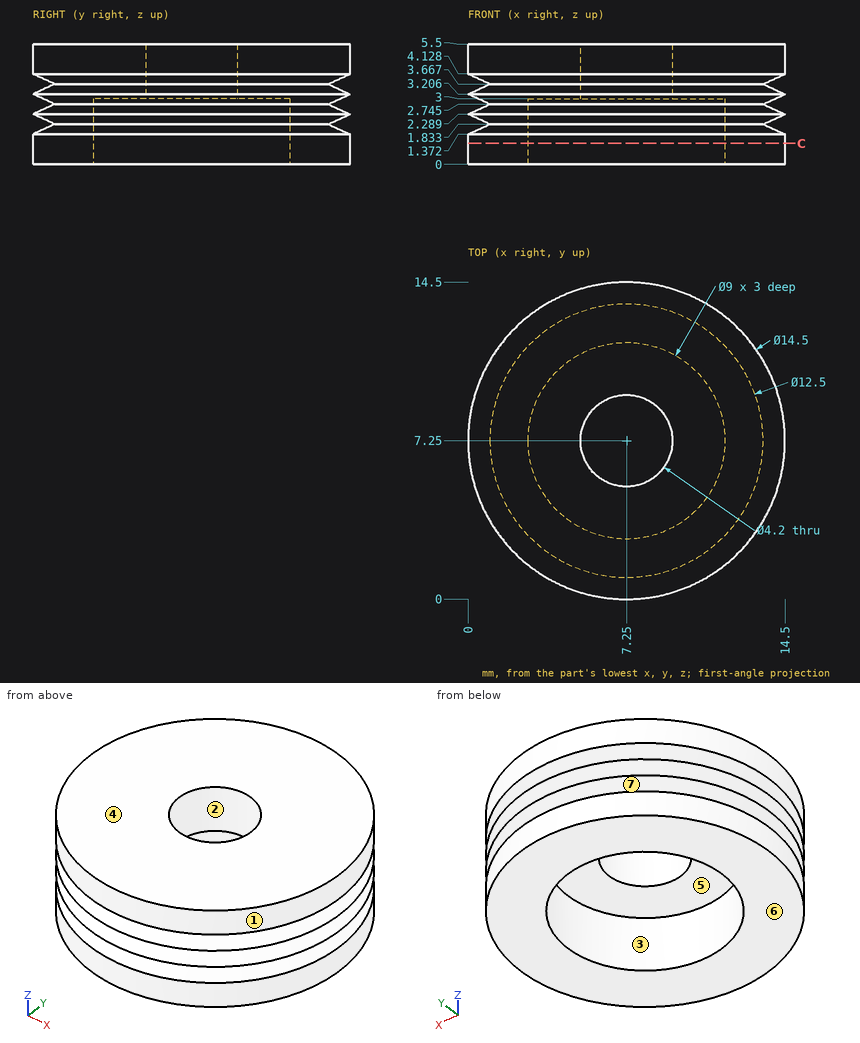
For this review, use the dimensioned drawing (mm, ordinates from the lowest corner) and the shaded views. A direction names the side the tool comes from. Give positions to 0.01 mm unless a question says otherwise; leave off trailing zeros. Order: outer loops, then holes, each group sorted by start corner. A loop starts at its lowest first (then second) coordinate and runs counter-clockwise, first axis right, second up. Notation, with made-up numbers: M 39,27 L 83,27 A23 ccw 83,52 Z; hole C 76.5,63.5 d7. An arc over 180 degrees is marked long. Use one line per item in the form item = value. Start each with the question number.
Item 1: The part is to be moulded in two halves that separate along Y. For the marked faces 1, 2, 3 and 4, say which applies: pulls with the +Y half, pulls with the -Y half, needs draft (parallel to the pull), parting line crosses it, or undercut.
Item 2: Insertion check: pin 1 Ø3 at (x, y) = (2, 3) entering from -Z; pin 2 Ø1.5 at (y, z) = (13, 1.5) entering from -X; pin 3 Ø2.5 at (x, y) = (7, 8.5) entering from -Z. Each pin has a flat end and moves straight along its axis. Give the tip position at first contact, or say it passes through.
Item 3: We need section C-C on z = 0.95. Give the boundary of the cut face in (x, y).
Item 4: To check wall thickness, follow line 1 along Y through (x, z) = (7.25, 4.2); line 2 along Z through (x, y) = (6.5, 4.25); line 3 along Z through (x, y) = (2.25, 3) (1 decimal). State the ranges of each line that lie inside material, in increasing order. Write a range as from..to.
Item 5: For the marked faces 5, 6 and 7, list the 3-axis set-ups (+Z, -Z, +X, -X, +Y, -Y) from which the entire face can be reached by the end or side of a thin tool; tool diameter is ignored.
Completed:
q1.face_1 = parting line crosses it
q1.face_2 = undercut
q1.face_3 = undercut
q1.face_4 = needs draft
q2.pin_1 = 0
q2.pin_2 = 2.01
q2.pin_3 = 3
q3.outline = C 7.25,7.25 d14.5; hole C 7.25,7.25 d9
q4.line_1 = 0..5.15, 9.35..14.5
q4.line_2 = 3..5.5
q4.line_3 = 0..1.7, 2..2.6, 2.9..3.5, 3.8..5.5
q5.face_5 = -Z
q5.face_6 = -Z, +X, -X, +Y, -Y
q5.face_7 = none
